CAD build for the part. Positions are in the model's coordinates, mm. Coordinates: 2 decimals unless noted, no trailing zeros. Order: outer loops, then holes, each group sorted by start corner. A loop starts at its lowest first (then second) coordinate and runs counter-clockwise, first axis right, second up. Notation, with made-up numbers: M 84,-4 L 111,-4 A17 ccw 111,9 Z; hole C 81.25,-4 d11. An arc over 180 degrees is marked long. Write item = value, one per line.
from build123d import *

# Parameters (mm, degrees)
ESQUISSE1_R             = 150
ESQUISSE1_R_2           = 100
BOSS_EXTRU_1_DEPTH      = 12
ESQUISSE2_R             = 17.5
BOSS_EXTRU_2_DEPTH      = 12
ESQUISSE3_R             = 10.5
BOSS_EXTRU_3_DEPTH      = 9
BOSS_EXTRU_4_DEPTH      = 12
BOSS_EXTRU_5_DEPTH      = 12
ENL_V_MAT_EXTRU_1_DEPTH = 274.749885845
ESQUISSE7_W             = 331.776450303
ESQUISSE7_H             = 53.126777449
ENL_V_MAT_EXTRU_2_DEPTH = 286
ESQUISSE8_R             = 12
ENL_V_MAT_EXTRU_3_DEPTH = 286
ENL_V_START             = 12
ENL_V_MAT_EXTRU_5_DEPTH = 4
ESQUISSE11_R            = 2
ENL_V_MAT_EXTRU_6_DEPTH = 10


with BuildPart() as part:
    # Esquisse1 → Boss.-Extru.1 (new body)
    with BuildSketch(Plane.XY):
        Circle(ESQUISSE1_R)
        Circle(ESQUISSE1_R_2, mode=Mode.SUBTRACT)
    extrude(amount=BOSS_EXTRU_1_DEPTH)

    # Esquisse2 → Boss.-Extru.2 (add)
    with BuildSketch(Plane.XY.offset(12)):
        with Locations((0, 125)):
            Circle(ESQUISSE2_R)
        with Locations((73.473156537, 101.127124297)):
            Circle(ESQUISSE2_R)
        with Locations((118.882064537, 38.627124297)):
            Circle(ESQUISSE2_R)
        with Locations((118.882064537, -38.627124297)):
            Circle(ESQUISSE2_R)
        with Locations((73.473156537, -101.127124297)):
            Circle(ESQUISSE2_R)
        with Locations((0, -125)):
            Circle(ESQUISSE2_R)
        with Locations((-73.473156537, -101.127124297)):
            Circle(ESQUISSE2_R)
        with Locations((-118.882064537, -38.627124297)):
            Circle(ESQUISSE2_R)
        with Locations((-118.882064537, 38.627124297)):
            Circle(ESQUISSE2_R)
        with Locations((-73.473156537, 101.127124297)):
            Circle(ESQUISSE2_R)
    extrude(amount=BOSS_EXTRU_2_DEPTH)

    # Esquisse3 → Boss.-Extru.3 (add)
    with BuildSketch(Plane.XY.offset(24)):
        with Locations((0, 125)):
            Circle(ESQUISSE3_R)
        with Locations((73.473156537, 101.127124297)):
            Circle(ESQUISSE3_R)
        with Locations((118.882064537, 38.627124297)):
            Circle(ESQUISSE3_R)
        with Locations((118.882064537, -38.627124297)):
            Circle(ESQUISSE3_R)
        with Locations((73.473156537, -101.127124297)):
            Circle(ESQUISSE3_R)
        with Locations((0, -125)):
            Circle(ESQUISSE3_R)
        with Locations((-73.473156537, -101.127124297)):
            Circle(ESQUISSE3_R)
        with Locations((-118.882064537, -38.627124297)):
            Circle(ESQUISSE3_R)
        with Locations((-118.882064537, 38.627124297)):
            Circle(ESQUISSE3_R)
        with Locations((-73.473156537, 101.127124297)):
            Circle(ESQUISSE3_R)
    extrude(amount=BOSS_EXTRU_3_DEPTH)

    # Esquisse4 → Boss.-Extru.4 (add)
    # profile 1 of 4: a face of its own
    with BuildSketch(Plane.XY.offset(12)):
        with BuildLine():
            Line((-14, 145), (-14, 185))
            ThreePointArc((-14, 185), (-11.656854249, 190.656854249), (-6, 193))
            Line((-6, 193), (6, 193))
            ThreePointArc((6, 193), (11.656854249, 190.656854249), (14, 185))
            Line((14, 185), (14, 145))
            Line((14, 145), (-14, 145))
        make_face()
        with BuildLine():
            Line((-3.75, 154.53605372), (-3.75, 184.53605372))
            ThreePointArc((-3.75, 184.53605372), (0, 188.28605372), (3.75, 184.53605372))
            Line((3.75, 184.53605372), (3.75, 154.53605372))
            ThreePointArc((3.75, 154.53605372), (0, 150.78605372), (-3.75, 154.53605372))
        make_face(mode=Mode.SUBTRACT)
    # profile 2 of 4: a face of its own
    with BuildSketch(Plane.XY.offset(12)):
        with BuildLine():
            Line((145, 14), (145, -14))
            Line((145, -14), (185, -14))
            ThreePointArc((185, -14), (190.656854249, -11.656854249), (193, -6))
            Line((193, -6), (193, 6))
            ThreePointArc((193, 6), (190.656854249, 11.65685425), (185, 14))
            Line((185, 14), (145, 14))
        make_face()
        with BuildLine():
            Line((154.53605372, -3.75), (184.53605372, -3.75))
            ThreePointArc((184.53605372, -3.75), (188.28605372, 0), (184.53605372, 3.75))
            Line((184.53605372, 3.75), (154.53605372, 3.75))
            ThreePointArc((154.53605372, 3.75), (150.78605372, 0), (154.53605372, -3.75))
        make_face(mode=Mode.SUBTRACT)
    # profile 3 of 4: a face of its own
    with BuildSketch(Plane.XY.offset(12)):
        with BuildLine():
            Line((14, -145), (-14, -145))
            Line((-14, -145), (-14, -185))
            ThreePointArc((-14, -185), (-11.656854249, -190.656854249), (-6, -193))
            Line((-6, -193), (6, -193))
            ThreePointArc((6, -193), (11.656854249, -190.656854249), (14, -185))
            Line((14, -185), (14, -145))
        make_face()
        with BuildLine():
            Line((-3.75, -154.53605372), (-3.75, -184.53605372))
            ThreePointArc((-3.75, -184.53605372), (0, -188.28605372), (3.75, -184.53605372))
            Line((3.75, -184.53605372), (3.75, -154.53605372))
            ThreePointArc((3.75, -154.53605372), (0, -150.78605372), (-3.75, -154.53605372))
        make_face(mode=Mode.SUBTRACT)
    # profile 4 of 4: a face of its own
    with BuildSketch(Plane.XY.offset(12)):
        with BuildLine():
            Line((-145, -14), (-145, 14))
            Line((-145, 14), (-185, 14))
            ThreePointArc((-185, 14), (-190.656854249, 11.65685425), (-193, 6))
            Line((-193, 6), (-193, -6))
            ThreePointArc((-193, -6), (-190.656854249, -11.656854249), (-185, -14))
            Line((-185, -14), (-145, -14))
        make_face()
        with BuildLine():
            Line((-154.53605372, 3.75), (-184.53605372, 3.75))
            ThreePointArc((-184.53605372, 3.75), (-188.28605372, 0), (-184.53605372, -3.75))
            Line((-184.53605372, -3.75), (-154.53605372, -3.75))
            ThreePointArc((-154.53605372, -3.75), (-150.78605372, 0), (-154.53605372, 3.75))
        make_face(mode=Mode.SUBTRACT)
    extrude(amount=-BOSS_EXTRU_4_DEPTH)

    # Esquisse5 → Boss.-Extru.5 (add)
    with BuildSketch(Plane.XY.offset(12)):
        with BuildLine():
            Line((-6, 193), (6, 193))
            ThreePointArc((6, 193), (14.453112805, 191.014875198), (21.138947402, 185.474527528))
            Line((21.138947402, 185.474527528), (78.676319934, 122.506579561))
            Line((78.676319934, 122.506579561), (0, 146.402607913))
            Line((0, 146.402607913), (-78.676319934, 122.506579561))
            Line((-78.676319934, 122.506579561), (-21.138947402, 185.474527528))
            ThreePointArc((-21.138947402, 185.474527528), (-14.453112805, 191.014875198), (-6, 193))
        make_face()
        with BuildLine():
            Line((146.402607913, 0), (122.506579561, -78.676319934))
            Line((122.506579561, -78.676319934), (185.474527528, -21.138947402))
            ThreePointArc((185.474527528, -21.138947402), (191.014875198, -14.453112805), (193, -6))
            Line((193, -6), (193, 6))
            ThreePointArc((193, 6), (191.014875198, 14.453112805), (185.474527528, 21.138947402))
            Line((185.474527528, 21.138947402), (122.506579561, 78.676319934))
            Line((122.506579561, 78.676319934), (146.402607913, 0))
        make_face()
        with BuildLine():
            Line((0, -146.402607913), (-78.676319934, -122.506579561))
            Line((-78.676319934, -122.506579561), (-21.138947402, -185.474527528))
            ThreePointArc((-21.138947402, -185.474527528), (-14.453112805, -191.014875198), (-6, -193))
            Line((-6, -193), (6, -193))
            ThreePointArc((6, -193), (14.453112805, -191.014875198), (21.138947402, -185.474527528))
            Line((21.138947402, -185.474527528), (78.676319934, -122.506579561))
            Line((78.676319934, -122.506579561), (0, -146.402607913))
        make_face()
        with BuildLine():
            Line((-146.402607913, 0), (-122.506579561, 78.676319934))
            Line((-122.506579561, 78.676319934), (-185.474527528, 21.138947402))
            ThreePointArc((-185.474527528, 21.138947402), (-191.014875198, 14.453112805), (-193, 6))
            Line((-193, 6), (-193, -6))
            ThreePointArc((-193, -6), (-191.014875198, -14.453112805), (-185.474527528, -21.138947402))
            Line((-185.474527528, -21.138947402), (-122.506579561, -78.676319934))
            Line((-122.506579561, -78.676319934), (-146.402607913, 0))
        make_face()
    extrude(amount=-BOSS_EXTRU_5_DEPTH)

    # Esquisse6 → Enlèv. mat.-Extru.1 (cut, through all)
    with BuildSketch(Plane.XY.offset(12)):
        with BuildLine():
            Line((-3.5, 157.595940505), (-3.5, 173.595940505))
            ThreePointArc((-3.5, 173.595940505), (0, 177.095940505), (3.5, 173.595940505))
            Line((3.5, 173.595940505), (3.5, 157.595940505))
            ThreePointArc((3.5, 157.595940505), (0, 154.095940505), (-3.5, 157.595940505))
        make_face()
        with BuildLine():
            Line((161.329273839, -7.233333333), (177.329273839, -7.233333333))
            ThreePointArc((177.329273839, -7.233333333), (180.829273839, -3.733333333), (177.329273839, -0.233333333))
            Line((177.329273839, -0.233333333), (161.329273839, -0.233333333))
            ThreePointArc((161.329273839, -0.233333333), (157.829273839, -3.733333333), (161.329273839, -7.233333333))
        make_face()
        with BuildLine():
            Line((-3.5, -165.062607172), (-3.5, -181.062607172))
            ThreePointArc((-3.5, -181.062607172), (0, -184.562607172), (3.5, -181.062607172))
            Line((3.5, -181.062607172), (3.5, -165.062607172))
            ThreePointArc((3.5, -165.062607172), (0, -161.562607172), (-3.5, -165.062607172))
        make_face()
        with BuildLine():
            Line((-161.329273838, -0.233333333), (-177.329273838, -0.233333333))
            ThreePointArc((-177.329273838, -0.233333333), (-180.829273838, -3.733333333), (-177.329273838, -7.233333333))
            Line((-177.329273838, -7.233333333), (-161.329273838, -7.233333333))
            ThreePointArc((-161.329273838, -7.233333333), (-157.829273838, -3.733333333), (-161.329273838, -0.233333333))
        make_face()
    extrude(amount=-ENL_V_MAT_EXTRU_1_DEPTH, mode=Mode.SUBTRACT)

    # Esquisse7 → Enlèv. mat.-Extru.2 (cut, symmetric)
    with BuildSketch(Plane(origin=(0, 0, 0), x_dir=(1, 0, 0), z_dir=(0, 1, 0))):
        with Locations((9.877314169, -38.563388725)):
            Rectangle(ESQUISSE7_W, ESQUISSE7_H)
    extrude(amount=ENL_V_MAT_EXTRU_2_DEPTH, both=True, mode=Mode.SUBTRACT)

    # Esquisse8 → Enlèv. mat.-Extru.3 (cut, symmetric)
    with BuildSketch(Plane.XY.offset(12)):
        with Locations((81.317279836, 81.317279836)):
            Circle(ESQUISSE8_R)
        with Locations((-81.317279836, 81.317279836)):
            Circle(ESQUISSE8_R)
        with Locations((81.317279836, -81.317279836)):
            Circle(ESQUISSE8_R)
        with Locations((-81.317279836, -81.317279836)):
            Circle(ESQUISSE8_R)
    extrude(amount=ENL_V_MAT_EXTRU_3_DEPTH, both=True, mode=Mode.SUBTRACT)

    # Esquisse10 → Enlèv. mat.-Extru.5 (cut)
    with BuildSketch(Plane.XY.offset(ENL_V_START)):
        Polygon((-65.707736407, 94.76323817), (-61.720728388, 92.431479094), (-57.707861783, 94.718449786), (-57.682003198, 99.337179554), (-61.669011217, 101.668938629), (-65.681877822, 99.381967937), align=None)
        Polygon((-101.668938629, -61.669011217), (-99.381967937, -65.681877822), (-94.76323817, -65.707736407), (-92.431479094, -61.720728388), (-94.718449786, -57.707861783), (-99.337179554, -57.682003198), align=None)
        Polygon((-57.076140035, -97.076067447), (-59.363110727, -93.063200842), (-63.981840494, -93.037342257), (-66.31359957, -97.024350276), (-64.026628878, -101.037216881), (-59.40789911, -101.063075466), align=None)
        Polygon((-101.037216881, 64.026628878), (-101.063075466, 59.40789911), (-97.076067447, 57.076140035), (-93.063200842, 59.363110727), (-93.037342257, 63.981840494), (-97.024350276, 66.31359957), align=None)
        Polygon((94.76323817, 65.707736407), (92.431479094, 61.720728388), (94.718449786, 57.707861783), (99.337179554, 57.682003198), (101.668938629, 61.669011217), (99.381967937, 65.681877822), align=None)
        Polygon((64.026628878, 101.037216881), (59.40789911, 101.063075466), (57.076140035, 97.076067447), (59.363110727, 93.063200842), (63.981840494, 93.037342257), (66.31359957, 97.024350276), align=None)
        Polygon((65.707736407, -94.76323817), (61.720728388, -92.431479094), (57.707861783, -94.718449786), (57.682003198, -99.337179554), (61.669011217, -101.668938629), (65.681877822, -99.381967937), align=None)
        Polygon((101.037216881, -64.026628878), (101.063075466, -59.40789911), (97.076067447, -57.076140035), (93.063200842, -59.363110727), (93.037342257, -63.981840494), (97.024350276, -66.31359957), align=None)
    extrude(amount=-ENL_V_MAT_EXTRU_5_DEPTH, mode=Mode.SUBTRACT)

    # Esquisse11 → Enlèv. mat.-Extru.6 (cut)
    with BuildSketch(Plane.XY):
        with Locations((-97.050208862, -61.694869802)):
            Circle(ESQUISSE11_R)
        with Locations((-61.694869802, -97.050208862)):
            Circle(ESQUISSE11_R)
        with Locations((-61.694869802, 97.050208862)):
            Circle(ESQUISSE11_R)
        with Locations((-97.050208862, 61.694869802)):
            Circle(ESQUISSE11_R)
        with Locations((97.050208862, 61.694869802)):
            Circle(ESQUISSE11_R)
        with Locations((61.694869802, 97.050208862)):
            Circle(ESQUISSE11_R)
        with Locations((61.694869802, -97.050208862)):
            Circle(ESQUISSE11_R)
        with Locations((97.050208862, -61.694869802)):
            Circle(ESQUISSE11_R)
    extrude(amount=ENL_V_MAT_EXTRU_6_DEPTH, mode=Mode.SUBTRACT)


solid = part.part
(1) Pull direction Y, two halves, no side cores. Call faces 1 (the face through (-159.738, -44.656, 6.084)), 2 (the face through (-159.01, 45.32, 6.08)), 3 (the face through (169, -0.233, 6)), 4 (the face through (-3.5, -173, 6)): +Y half, -Y half, draft (parallel to the pull), parting line (faces both ways), or undercut.
Evaluation:
face_1 = -Y half
face_2 = +Y half
face_3 = undercut
face_4 = undercut
(2) Pin check, flat tips, straight feed: pin 1 Ø2.5 at (x, y) = (63, -95.5) entering from +Z; pin 2 Ø19 at (x, y) = (-81.32, 81.32) entering from -Z; pin 3 Ø4 at (x, y) = (59.5, 96.5) entering from +Z; pin 4 Ø6 at (y, z) = (-174.5, 4.5) entering from -X. Stop position of each tip, or through.
Evaluation:
pin_1 = 8
pin_2 = through
pin_3 = 12
pin_4 = -33.91
(3) Slice it at D-D, the plane x = 166.5. Write the cut outline in (y, z).
Evaluation:
outline = M -38.48,0 L -7.23,0 L -7.23,12 L -38.48,12 Z; M -0.23,0 L 38.48,0 L 38.48,12 L -0.23,12 Z
(4) Slice it at C-C, the plane z = 4. State how many separate pieces and enclosed holes the cut face has, then the cut area to 3 significant figures.
Evaluation:
separate_pieces = 1
enclosed_holes = 17
area = 50,300 mm²
(5) Slice it at B-B, the plane x = -88. Write the cut outline in (y, z).
Evaluation:
outline = M -121.47,0 L -91.28,0 L -91.28,12 L -121.47,12 Z; M -71.35,0 L -47.5,0 L -47.5,12 L -71.35,12 Z; M 47.5,0 L 71.35,0 L 71.35,12 L 47.5,12 Z; M 91.28,0 L 121.47,0 L 121.47,12 L 91.28,12 Z
(6) Slice it at A-A, the plane x = 29. Write the cut outline in (y, z).
Evaluation:
outline = M -176.87,0 L -95.7,0 L -95.7,12 L -176.87,12 Z; M 95.7,0 L 176.87,0 L 176.87,12 L 95.7,12 Z
(7) Wall check: line 1 (Y direction, x = 0, z = 5.25); line 2 (Y direction, x = -74, z = 8.75); line 3 (X direction, y = -63, z = 4). Give the ranges that are in metal, low to high. Write a range as from..to.
Evaluation:
line_1 = -193..-184.56, -161.56..-100, 100..154.1, 177.1..193
line_2 = -130.48..-90.83, -71.81..-67.26, 67.26..71.81, 90.83..130.48
line_3 = -139.66..-98.57, -95.53..-77.66, 77.66..95.53, 98.57..139.66
